CAD build for the part. Positions are in the model's coordinates, mm. Coordinates: 2 decimals unless noted, no trailing zeros. Order: outer loops, then holes, each group sorted by start corner. A loop starts at its lowest first (then second) coordinate and runs counter-clockwise, first axis right, second up. Notation, with made-up numbers: (-16, 37) - (23, 37) arc R24 cw to (23, 72) - close; hole circle Ø8 at (48.5, 77). An arc over 180 degrees is marked (long way). Use one line per item in the form item = value.
Autodesk Inventor part; units mm, degrees
ref_plane "YZ Plane" through (0, 0, 0) normal (1, 0, 0) x (0, 1, 0)
ref_plane "XZ Plane" through (0, 0, 0) normal (0, 1, 0) x (-1, 0, 0)
ref_plane "XY Plane" through (0, 0, 0) normal (0, 0, 1) x (1, 0, 0)
sketch "Skizze1" plane through (0, 0, 0) normal (0, 0, 1) x (1, 0, 0)
  line L0 (-36.3412, 23.6948) -> (23.6588, 23.6948)
  line L1 (23.6588, 23.6948) -> (23.6588, -16.3052)
  line L2 (23.6588, -16.3052) -> (-36.3412, -16.3052)
  line L3 (-36.3412, -16.3052) -> (-36.3412, 23.6948)
  point P0 (0, 0)
  dimension "d0" = 60
  dimension "d1" = 40
extrude "Extrusion1" add sketch "Skizze1" along normal blind 10
chamfer "Fase1" distance 9 angle 45 1 edges at (23.6588, 3.6948, 0)
fillet "Rundung1" radius 2 2 edges at (23.6588, 3.6948, 9) (14.6588, 3.6948, 0)
properties part number "KabelBoxDeckel"
Item 1: Two-plate mould, pull along X, no slides. Class faces 1 (the face through (23.5, 3.41, 9.05)), 2 (the face through (-7, 23.695, 5)), 3 (the face through (-36.341, 3, 5)): +X half, -X half, draft (parallel to the pull), parting line (faces both ways), or undercut.
Derived:
face_1 = +X half
face_2 = draft
face_3 = -X half
Item 2: Cut at A-A, the plane y = 2. Write the cut outline in (x, z), plus the area to 3 significant figures.
Derived:
outline = (-36.34, 0) - (13.83, 0) arc R2 ccw to (15.24, 0.59) - (23.07, 8.41) arc R2 ccw to (23.66, 9.83) - (23.66, 10) - (-36.34, 10) - close
area = 559 mm²
Item 3: Drill centre lines: line 1 (X direction, y = 11, z = 4.75); line 2 (X direction, y = 13, z = 0.5); line 3 (Z direction, x = 19, y = 15.5). Where is each one in solid material? Low to high. Write a range as [from, to].
Derived:
line_1 = [-36.34, 19.41]
line_2 = [-36.34, 15.15]
line_3 = [4.34, 10]
Item 4: Cut at C-C, the plane z = 2.5. Write the cut outline in (x, y).
Derived:
outline = (-36.34, -16.31) - (17.16, -16.31) - (17.16, 23.69) - (-36.34, 23.69) - close
Item 5: Cut at B-B, the plane z = 7. Write the cut outline in (x, y).
Derived:
outline = (-36.34, -16.31) - (21.66, -16.31) - (21.66, 23.69) - (-36.34, 23.69) - close
